from build123d import *

# Parameters (mm, degrees)
F1_DEPTH = 12.7
F2_R     = 1.905
F3_DEPTH = 10.16


with BuildPart() as f1:
    # F0 (on Front) → F1 (new body)
    with BuildSketch(Plane.XZ):
        Polygon((0, 8.854078), (0, 1.234078), (22.86, 1.234078), (22.86, 8.854078), (16.271867, 8.854078), (10.847912, 8.854078), (5.423956, 8.854078), align=None)
        Polygon((5.423956, 12.156078), (0, 8.854078), (5.423956, 8.854078), align=None)
        Polygon((10.847912, 12.156078), (5.423956, 8.854078), (10.847912, 8.854078), align=None)
        Polygon((10.847912, 8.854078), (16.271867, 8.854078), (16.271867, 12.156078), align=None)
    extrude(amount=F1_DEPTH)

    # F2 (on face) → F3 (join)
    with BuildSketch(Plane.XY.offset(8.854078)):
        with Locations((19.685, -3.175)):
            Circle(F2_R)
        with Locations((19.685, -9.525)):
            Circle(F2_R)
    extrude(amount=F3_DEPTH)


solid = f1.part
Can you work these out from the model? Positions are in its coordinate system, mm. A direction names the side the tool comes from. Coordinates: 2 decimals unless noted, no trailing zeros. Order: outer loops, then holes, each group sorted by start corner. A loop starts at its lowest first (then second) coordinate and runs counter-clockwise, first axis right, second up. Notation, with made-up numbers: (43.25, -28) -> (89.25, -28) arc R25 ccw to (89.25, -7) -> close; hole circle Ø9 at (-18, 70.25). An arc over 180 degrees is marked (long way). Use one line per item in the form item = value.
Q1. Which directions (+Z, -Z, +X, -X, +Y, -Y) give clear straight access to the entire face, cutting with the end or side of a thin tool? Please do faces 1 (the face through (20, -9, 19.014)), 2 (the face through (16.272, -6, 10)), 3 (the face through (20, -6, 8.854)).
From the geometry:
face_1 = +Z, +X, -X, +Y, -Y
face_2 = +Z, +Y, -Y
face_3 = +Z
Q2. Imagine slicing it at A-A, the plane y = -7. List the corners of the cut face in (x, z) for me, then the cut area to 3 significant figures.
From the geometry:
outline = (0, 1.23) -> (22.86, 1.23) -> (22.86, 8.85) -> (16.27, 8.85) -> (16.27, 12.16) -> (10.85, 8.85) -> (10.85, 12.16) -> (5.42, 8.85) -> (5.42, 12.16) -> (0, 8.85) -> close
area = 201 mm²
Q3. Imagine slicing it at D-D, the plane z = 18. List the corners of the cut face in (x, y) for me (3 decimals), then the cut area to 3 significant figures.
From the geometry:
outline = circle Ø3.81 at (19.685, -9.525); circle Ø3.81 at (19.685, -3.175)
area = 22.8 mm²
Q4. We'd pull the mould along X, two halves only. Please class faces 4 (the face through (13.6, -6.26, 10.53)), 5 (the face through (20, -3, 19.014)), 6 (the face through (2.7, -6.3, 10.5)): released by +X, released by -X, zero draft, split by the parting line, or undercut.
From the geometry:
face_4 = undercut
face_5 = zero draft
face_6 = released by -X
Q5. I need wall thicknesses on L1, parallel to X at y = -4, z = 9; L2, parallel to X at y = -3.25, z = 18.25; L3, parallel to X at y = -1.5, z = 14.25. Which ranges of each line are inside material? Lowest first, please.
From the geometry:
L1 = 0.24 to 5.42, 5.66 to 10.85, 11.09 to 16.27, 17.97 to 21.4
L2 = 17.78 to 21.59
L3 = 18.78 to 20.59
Q6. Will these pins go through, and if not, where does the flat tip stop? P1, Ø1, axis at y = -4.5, z = 11, coming from the +X side; P2, Ø1.7, axis at y = -5, z = 11.5, coming from the +X side; P3, Ø3, axis at x = 18.5, z = 11, coming from the -Y side.
From the geometry:
P1 = 21.4
P2 = 21.32
P3 = -11.43
Q7. Imagine slicing it at B-B, the plane z = 10. List the corners of the cut face in (x, y) for me (3 decimals), then the cut area to 3 significant figures.
From the geometry:
outline = (1.882, -12.7) -> (5.424, -12.7) -> (5.424, 0) -> (1.882, 0) -> close; (7.306, -12.7) -> (10.848, -12.7) -> (10.848, 0) -> (7.306, 0) -> close; (12.73, -12.7) -> (16.272, -12.7) -> (16.272, 0) -> (12.73, 0) -> close; circle Ø3.81 at (19.685, -9.525); circle Ø3.81 at (19.685, -3.175)
area = 158 mm²
Q8. Imagine slicing it at C-C, the plane x = 21. List the corners of the cut face in (y, z) for me.
From the geometry:
outline = (-12.7, 1.23) -> (0, 1.23) -> (0, 8.85) -> (-1.8, 8.85) -> (-1.8, 19.01) -> (-4.55, 19.01) -> (-4.55, 8.85) -> (-8.15, 8.85) -> (-8.15, 19.01) -> (-10.9, 19.01) -> (-10.9, 8.85) -> (-12.7, 8.85) -> close
